The drawing under review shows one solid part. Ordinate dimensions are in mm from its lowest x, y, z. Round coordinates to 2 decimals unless told otherwise and drop trailing zeros. Order: outer loops, then holes, each group sorted by start corner. A loop starts at its lowest first (then second) coordinate and runs counter-clockwise, first axis right, second up. Notation, with made-up numbers: (-3, -12) - (30, -12) arc R19 ccw to (30, 8) - close; hole circle Ø11 at (24.5, -33). An arc over 180 degrees is marked (long way). One line per question, with ' | ' between items.
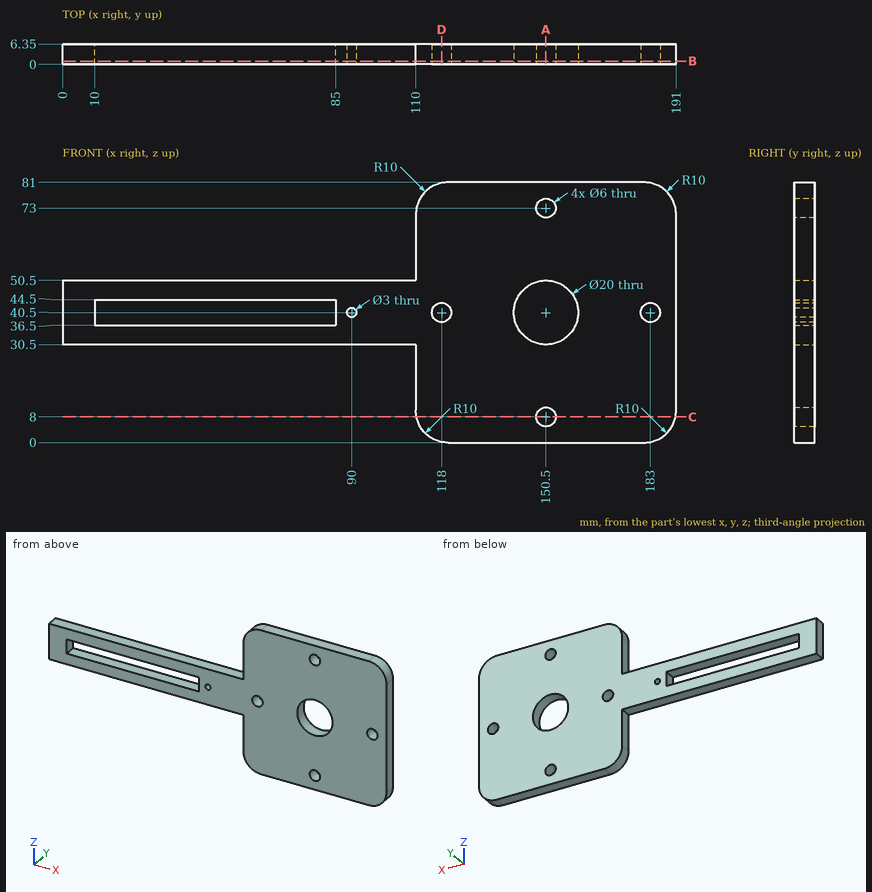
(1) We need section A-A on x = 150.5. State the section outline as (y, z) points.
Output values:
outline: (0, 0) - (6.35, 0) - (6.35, 5) - (0, 5) - close; (0, 11) - (6.35, 11) - (6.35, 30.5) - (0, 30.5) - close; (0, 50.5) - (6.35, 50.5) - (6.35, 70) - (0, 70) - close; (0, 76) - (6.35, 76) - (6.35, 81) - (0, 81) - close
(2) For probe 1 along X at (y, z) = (4.75, 40.5); probe 2 along Z at (x, y) = (84, 1.75); probe 3 along Z at (x, y) = (90, 2.75), list the stretches that pass through material, from the lowest coordinate up. Write a range as [from, to].
Output values:
probe 1: [0, 10], [85, 88.5], [91.5, 115], [121, 140.5], [160.5, 180], [186, 191] | probe 2: [30.5, 36.5], [44.5, 50.5] | probe 3: [30.5, 39], [42, 50.5]
(3) Insertion check: pin 1 (3.5 mm diameter, centred on x = 118, z = 40.5, fed in from +Y); pin 2 (9.5 mm diameter, centred on x = 150.5, z = 8, fed in from +Y); pin 3 (1.9 mm diameter, centred on x = 34.5, y = 4.5, fed in from +Z); pin 4 (1.9 mm diameter, centred on x = 59.5, y = 4, fed in from -Z). Each pin has a flat end and moves straight along its axis. Give the tip position at first contact, or say it passes through.
Output values:
pin 1: through | pin 2: y = 6.35 | pin 3: z = 50.5 | pin 4: z = 30.5
(4) We need section D-D on x = 118. State the section outline as (y, z) points, plus the area to 3 significant figures.
Output values:
outline: (0, 0.2) - (6.35, 0.2) - (6.35, 37.5) - (0, 37.5) - close; (0, 43.5) - (6.35, 43.5) - (6.35, 80.8) - (0, 80.8) - close | area: 474 mm^2
(5) We need section B-B on y = 1. State the section outline as (x, z) points.
Output values:
outline: (0, 30.5) - (110, 30.5) - (110, 10) arc R10 ccw to (120, 0) - (181, 0) arc R10 ccw to (191, 10) - (191, 71) arc R10 ccw to (181, 81) - (120, 81) arc R10 ccw to (110, 71) - (110, 50.5) - (0, 50.5) - close; hole (10, 36.5) - (85, 36.5) - (85, 44.5) - (10, 44.5) - close; hole circle Ø3 at (90, 40.5); hole circle Ø6 at (118, 40.5); hole circle Ø20 at (150.5, 40.5); hole circle Ø6 at (150.5, 8); hole circle Ø6 at (150.5, 73); hole circle Ø6 at (183, 40.5)
(6) We need section C-C on z = 8. State the section outline as (x, y) points, plus the area to 3 significant figures.
Output values:
outline: (110.2, 0) - (147.5, 0) - (147.5, 6.35) - (110.2, 6.35) - close; (153.5, 0) - (190.8, 0) - (190.8, 6.35) - (153.5, 6.35) - close | area: 474 mm^2
